```python
from build123d import *

# Parameters (mm, degrees)
F0_W     = 1.5
F0_H     = 9.3130898729
F0_H_2   = 25.6233112887
F0_H_3   = 5.8635988384
F0_W_2   = 14
F0_H_4   = 2
F0_H_5   = 0.4158456028
F0_W_3   = 0.7
F0_W_4   = 0.5
F0_W_5   = 37.8
F0_H_6   = 8.5
F0_W_6   = 10
F0_H_7   = 1.5
F1_DEPTH = 2
F2_START = 1
F2_DEPTH = 3.5
F3_START = 3
F3_DEPTH = 1
F4_SIZE  = 0.49999


# Not quite as in the source:
# - a fillet or chamfer is up to 0.001 mm smaller than in the source, because OpenCascade refuses the exact size
# - a feature names something its author has since deleted; it is built from what else it names


with BuildPart() as f1:
    # F0 (on Top) → F1 (new body)
    with BuildSketch(Plane.XY):
        Polygon((-20.5, 25.9721875068), (-20.5, 35.9721875068), (20.3, 35.9721875068), (20.3, 25.9721875068), (20.8, 25.9721875068), (20.8, 16.6590976339), (20.3, 16.6590976339), (20.3, -8.9642136547), (21, -8.9642136547), (21, -14.8278124932), (20.3, -14.8278124932), (20.3, -24.8278124932), (17, -24.8278124932), (17, -26.8278124932), (22.3, -26.8278124932), (22.3, -13.9410611472), (22.3, 25.0854361609), (22.3, 37.9721875068), (-22.5, 37.9721875068), (-22.5, 25.0854361609), (-22.5, -13.9410611472), (-22.5, -26.8278124932), (-17, -26.8278124932), (-17, -24.8278124932), (-20.5, -24.8278124932), (-20.5, -14.8278124932), (-21, -14.8278124932), (-21, -8.9642136547), (-20.5, -8.9642136547), (-20.5, 16.6590976339), (-21, 16.6590976339), (-21, 25.9721875068), align=None)
        Polygon((20.3, 35.9721875068), (-20.5, 35.9721875068), (-20.5, 25.9721875068), (-19, 25.9721875068), (-19, 34.4721875068), (18.8, 34.4721875068), (18.8, 25.9721875068), (20.3, 25.9721875068), align=None)
        with Locations((-19.75, 21.3156425704)):
            Rectangle(F0_W, F0_H)
        with Locations((-19.75, 3.8474419896)):
            Rectangle(F0_W, F0_H_2)
        Polygon((18.8, -14.8278124932), (-19, -14.8278124932), (-19, -23.3278124932), (-7, -23.3278124932), (-7, -22.9119668904), (7, -22.9119668904), (7, -23.3278124932), (18.8, -23.3278124932), align=None)
        with Locations((-19.75, -11.8960130739)):
            Rectangle(F0_W, F0_H_3)
        with Locations((0, -25.8278124932)):
            Rectangle(F0_W_2, F0_H_4)
        with Locations((0, -23.1198896918)):
            Rectangle(F0_W_2, F0_H_5)
        Polygon((-19, -14.8278124932), (-20.5, -14.8278124932), (-20.5, -24.8278124932), (-17, -24.8278124932), (-7, -24.8278124932), (-7, -23.3278124932), (-19, -23.3278124932), align=None)
        with Locations((20.65, -11.8960130739)):
            Rectangle(F0_W_3, F0_H_3)
        with Locations((-20.75, -11.8960130739)):
            Rectangle(F0_W_4, F0_H_3)
        with Locations((-20.75, 21.3156425704)):
            Rectangle(F0_W_4, F0_H)
        with Locations((20.55, 21.3156425704)):
            Rectangle(F0_W_4, F0_H)
        with Locations((-0.1, 30.2221875068)):
            Rectangle(F0_W_5, F0_H_6)
        with Locations((-0.1, 21.3156425704)):
            Rectangle(F0_W_5, F0_H)
        with Locations((-0.1, 3.8474419896)):
            Rectangle(F0_W_5, F0_H_2)
        with Locations((-0.1, -11.8960130739)):
            Rectangle(F0_W_5, F0_H_3)
        with Locations((-12, -25.8278124932)):
            Rectangle(F0_W_6, F0_H_4)
        with Locations((0, -24.0778124932)):
            Rectangle(F0_W_2, F0_H_7)
        Polygon((20.3, -24.8278124932), (20.3, -14.8278124932), (18.8, -14.8278124932), (18.8, -23.3278124932), (7, -23.3278124932), (7, -24.8278124932), (17, -24.8278124932), align=None)
        with Locations((12, -25.8278124932)):
            Rectangle(F0_W_6, F0_H_4)
        with Locations((19.55, -11.8960130739)):
            Rectangle(F0_W, F0_H_3)
        with Locations((19.55, 3.8474419896)):
            Rectangle(F0_W, F0_H_2)
        with Locations((19.55, 21.3156425704)):
            Rectangle(F0_W, F0_H)
    extrude(amount=F1_DEPTH)

    # F0 (on Top) → F2 (join)
    with BuildSketch(Plane.XY.offset(F2_START)):
        Polygon((20.3, 35.9721875068), (-20.5, 35.9721875068), (-20.5, 25.9721875068), (-19, 25.9721875068), (-19, 34.4721875068), (18.8, 34.4721875068), (18.8, 25.9721875068), (20.3, 25.9721875068), align=None)
        with Locations((-19.75, 21.3156425704)):
            Rectangle(F0_W, F0_H)
        with Locations((-19.75, 3.8474419896)):
            Rectangle(F0_W, F0_H_2)
        with Locations((19.55, 21.3156425704)):
            Rectangle(F0_W, F0_H)
        with Locations((19.55, 3.8474419896)):
            Rectangle(F0_W, F0_H_2)
        Polygon((20.3, -24.8278124932), (20.3, -14.8278124932), (18.8, -14.8278124932), (18.8, -23.3278124932), (7, -23.3278124932), (7, -24.8278124932), (17, -24.8278124932), align=None)
        with Locations((19.55, -11.8960130739)):
            Rectangle(F0_W, F0_H_3)
        Polygon((-19, -14.8278124932), (-20.5, -14.8278124932), (-20.5, -24.8278124932), (-17, -24.8278124932), (-7, -24.8278124932), (-7, -23.3278124932), (-19, -23.3278124932), align=None)
        with Locations((-19.75, -11.8960130739)):
            Rectangle(F0_W, F0_H_3)
    extrude(amount=F2_DEPTH)

    # F0 (on Top) → F3 (join)
    with BuildSketch(Plane.XY.offset(F3_START)):
        with Locations((20.55, 21.3156425704)):
            Rectangle(F0_W_4, F0_H)
        with Locations((-20.75, 21.3156425704)):
            Rectangle(F0_W_4, F0_H)
        with Locations((-20.75, -11.8960130739)):
            Rectangle(F0_W_4, F0_H_3)
        with Locations((20.65, -11.8960130739)):
            Rectangle(F0_W_3, F0_H_3)
    extrude(amount=F3_DEPTH)

    # F4 (size 0.5 in the source; OpenCascade refuses exactly that, so slightly less here)
    f4_edges = [f1.edges().sort_by_distance(p)[0] for p in [
        (-21, 25.972188, 3.5),
        (-21, 16.659098, 3.5),
        (-21, 21.315643, 3),
        (-21, 21.315643, 4),
        (-21, -8.964214, 3.5),
        (-21, -14.827812, 3.5),
        (-21, -11.896013, 3),
        (-21, -11.896013, 4),
        (20.8, 16.659098, 3.5),
        (20.8, 25.972188, 3.5),
        (20.8, 21.315643, 3),
        (20.8, 21.315643, 4),
        (21, -14.827812, 3.5),
        (21, -8.964214, 3.5),
        (21, -11.896013, 3),
        (21, -11.896013, 4),
        (20.3, -24.827812, 3.25),
        (20.3, 35.972188, 3.25),
        (-0.1, 35.972188, 4.5),
        (-20.5, 5.572188, 4.5),
        (-13.75, -24.827812, 4.5),
        (-7, -24.077812, 4.5),
        (-13, -23.327812, 4.5),
        (-19, 5.572188, 4.5),
        (-0.1, 34.472188, 4.5),
        (18.8, 5.572188, 4.5),
        (12.9, -23.327812, 4.5),
        (7, -24.077812, 4.5),
        (13.65, -24.827812, 4.5),
        (20.3, 5.572188, 4.5),
        (-20.5, 35.972188, 3.25),
        (-22.5, 37.972188, 1),
        (-20.5, -24.827812, 3.25),
        (-22.5, -26.827812, 1),
        (22.3, -26.827812, 1),
        (22.3, 5.572188, 0),
        (-0.1, 37.972188, 0),
        (-22.5, 5.572188, 0),
        (-0.1, -26.827812, 0),
        (12.9, -23.327812, 2),
        (18.8, 5.572188, 2),
        (-13, -23.327812, 2),
        (-19, 5.572188, 2),
        (-0.1, 34.472188, 2),
        (7, -24.077812, 2),
        (-7, -24.077812, 2),
        (22.3, 37.972188, 1),
    ]]
    chamfer(f4_edges, length=F4_SIZE)


solid = f1.part
```
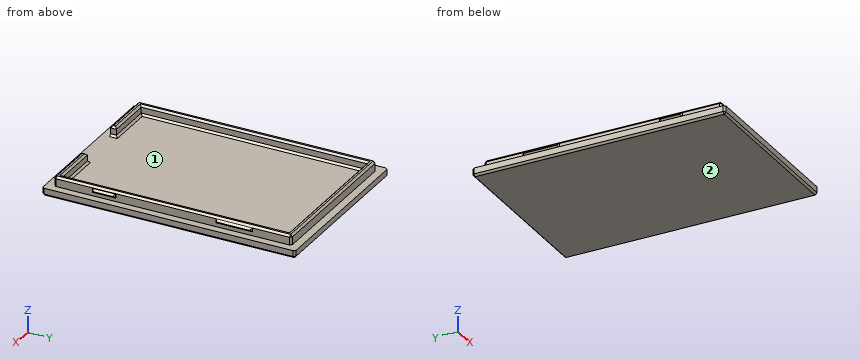
Read the model definition and answer for the solid it produces. Units are mm, in the model's axes. Face numbers are marked on the shaded views. Round coordinates to 2 decimals unless told otherwise and drop trailing zeros. Write each loop counter-clockwise with the first axis right and the second up, starting at its lowest first coordinate (ties: lowest second). Pieces come first, ordered by that corner, then holes. Notation, with made-up numbers: M 28,-37.5 L 60,-37.5 A22 cw 60,-12.5 Z; hole C 26,37 d4. An arc over 180 degrees is marked long. One line per item, written item: value.
Q1. Find section A-A on x = -5.5. Write down the section's boundary in (y, z).
Data:
outline: M -26.83,0.5 L -26.33,0 L 37.47,0 L 37.97,0.5 L 37.97,2 L 35.97,2 L 35.97,4 L 35.47,4.5 L 34.97,4.5 L 34.47,4 L 34.47,2.5 L 33.97,2 L -26.83,2 Z
Q2. Flat-ended cylindrical pins translate along their axes: pin 1 Ø1.5 at (x, z) = (13.5, 3.5) entering from -Y; pin 2 Ø1.2 at (y, z) = (-24, 3.5) entering from +X; pin 3 Ø1 at (y, z) = (19.5, 3.5) entering from +X. Find the tip coordinate at first contact, or state that the pin passes through.
Data:
pin 1: y = -24.83
pin 2: x = 20.3
pin 3: x = 20.8
Q3. Find section D-D on y = -20. Write down the section's boundary in (x, z).
Data:
outline: M -22.5,0.5 L -22,0 L 21.8,0 L 22.3,0.5 L 22.3,2 L 20.3,2 L 20.3,4 L 19.8,4.5 L 19.3,4.5 L 18.8,4 L 18.8,2.5 L 18.3,2 L -18.5,2 L -19,2.5 L -19,4 L -19.5,4.5 L -20,4.5 L -20.5,4 L -20.5,2 L -22.5,2 Z
Q4. Straight lines are drawn through the part: line 1 (Y direction, x = -8, z = 3.4); line 2 (X direction, y = 30, z = 3.8); line 3 (Z direction, x = 8, y = -6). For each, find the intervals that lie inside material, in ascending order. Write a range as [from, to].
Data:
line 1: [-24.83, -23.33], [34.47, 35.97]
line 2: [-20.5, -19], [18.8, 20.3]
line 3: [0, 2]
Q5. Find section C-C on x = 14.5. Write down the section's boundary in (y, z), plus the area to 3 significant figures.
Data:
outline: M -26.83,0.5 L -26.33,0 L 37.47,0 L 37.97,0.5 L 37.97,2 L 35.97,2 L 35.97,4 L 35.47,4.5 L 34.97,4.5 L 34.47,4 L 34.47,2.5 L 33.97,2 L -22.83,2 L -23.33,2.5 L -23.33,4 L -23.83,4.5 L -24.33,4.5 L -24.83,4 L -24.83,2 L -26.83,2 Z
area: 137 mm2
Q6. For a pull along X with two mould halves and no side action, classify the marked faces 1 and 2 as +X half, -X half, draft (parallel to the pull), parting line (faces both ways), or undercut.
Data:
face 1: undercut
face 2: draft
